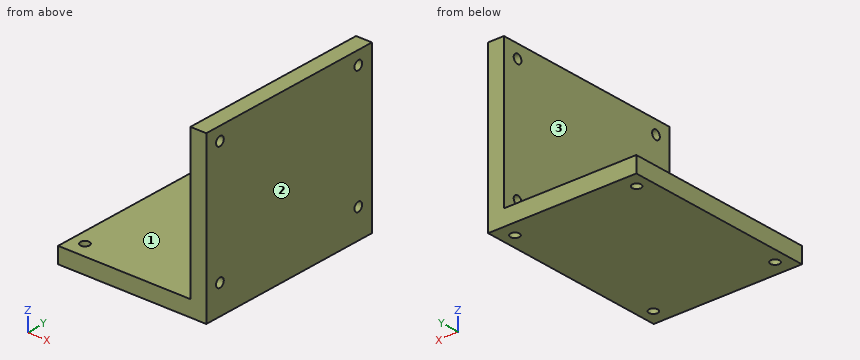
Solid Edge part; units mm, degrees
sketch "Sketch1" plane through (0, 0, 0) normal (0, 0, 1) x (1, 0, 0)
  line L0 (-28, -49) -> (28, -49)
  line L1 (28, -49) -> (28, 24)
  line L2 (28, 24) -> (-28, 24)
  line L3 (-28, 24) -> (-28, -49)
  circle A0 centre (-23, -43) radius 1.7
  circle A1 centre (23, -43) radius 1.7
  circle A2 centre (-23, 18) radius 1.7
  circle A3 centre (23, 18) radius 1.7
extrude "Protrusion1" add sketch "Sketch1" along normal blind 6
sketch "Sketch2" plane through (0, 0, 6) normal (0, 0, 1) x (1, 0, 0)
  line L0 (22, -49) -> (28, -49)
  line L1 (28, -49) -> (28, 24)
  line L2 (28, 24) -> (22, 24)
  line L3 (22, 24) -> (22, -49)
extrude "ExtrudedProtrusion_2" add sketch "Sketch2" along normal blind 56
sketch "Sketch3" plane through (22, 0, 0) normal (1, 0, 0) x (0, 1, 0)
  circle A0 centre (-43, 57) radius 1.7
  circle A1 centre (-43, 11) radius 1.7
  circle A2 centre (18, 57) radius 1.7
  circle A3 centre (18, 11) radius 1.7
extrude "ExtrudedCutout_1" cut sketch "Sketch3" along normal blind 6
Verification items for the finished model (mm, model axes). Face numbers are marked on the shaded views. Coordinates: 2 decimals unless noted, no trailing zeros. Loops run counter-clockwise (first coordinate to the right, second up) from the corner with the lowest first, then second, coordinate; pieces in that order, holes last. Notation, with made-up numbers: (56.25, -38.75) -> (102.25, -38.75) arc R13 ccw to (102.25, -25.75) -> close; hole circle Ø1 at (3.25, -14). An arc over 180 degrees is marked (long way). Answer in a Markdown table with one row per item.
1) Draft check along X on the marked faces 1, 2 and 3. Enter one of: released by +X, released by -X, zero draft, split by the parting line, or undercut.
The answers:
| item | result |
|---|---|
| face 1 | zero draft |
| face 2 | released by +X |
| face 3 | released by -X |
2) Section check B-B (x = -23). Record the cut outline in (y, z).
The answers:
| item | result |
|---|---|
| outline | (-49, 0) -> (-44.7, 0) -> (-44.7, 6) -> (-49, 6) -> close; (-41.3, 0) -> (16.3, 0) -> (16.3, 6) -> (-41.3, 6) -> close; (19.7, 0) -> (24, 0) -> (24, 6) -> (19.7, 6) -> close |
3) Scan lines: line 1 along Y through (x, z) = (-23, 1.4); line 2 along Z through (x, y) = (24, 16.5); line 3 along X through (y, z) = (-11, 15). Record each from-to range of solid material in increasing order. Write a range as from..to.
The answers:
| item | result |
|---|---|
| line 1 | y = -49..-44.7, -41.3..16.3, 19.7..24 |
| line 2 | z = 0..10.2, 11.8..56.2, 57.8..62 |
| line 3 | x = 22..28 |
4) Depth check by flat-ended pin: P1, Ø4, axis at x = -21, y = -27, coming from the +Z side; P2, Ø2.5, axis at x = -23, y = -43, coming from the -Z side; P3, Ø5.5, axis at y = -43, z = 57, coming from the -X side; P4, Ø0.8, axis at x = 23.5, y = 18.5, coming from the -Z side. Enter the tip coordinate at first touch or a pass-through.
The answers:
| item | result |
|---|---|
| P1 | stops at z = 6 |
| P2 | passes through |
| P3 | stops at x = 22 |
| P4 | stops at z = 6 |
5) Section check A-A (y = 18). Record the cut outline in (x, z).
The answers:
| item | result |
|---|---|
| outline | (-28, 0) -> (-24.7, 0) -> (-24.7, 6) -> (-28, 6) -> close; (-21.3, 0) -> (21.3, 0) -> (21.3, 6) -> (-21.3, 6) -> close; (22, 6) -> (24.7, 6) -> (24.7, 0) -> (28, 0) -> (28, 9.3) -> (22, 9.3) -> close; (22, 12.7) -> (28, 12.7) -> (28, 55.3) -> (22, 55.3) -> close; (22, 58.7) -> (28, 58.7) -> (28, 62) -> (22, 62) -> close |
6) Section check D-D (x = 11). Record the cut outline in (y, z).
The answers:
| item | result |
|---|---|
| outline | (-49, 0) -> (24, 0) -> (24, 6) -> (-49, 6) -> close |
7) Section check C-C (z = 51.5). Record the cut outline in (x, y), and give its area (3 significant figures).
The answers:
| item | result |
|---|---|
| outline | (22, -49) -> (28, -49) -> (28, 24) -> (22, 24) -> close |
| area | 438 mm2 |
